Model file for the job. Use its own axes, mm. Face numbers are marked on the shaded views. A direction names the side the tool comes from. Round coordinates to 2 decimals unless told otherwise and drop trailing zeros. Order: outer loops, then holes, each group sorted by start corner. A loop starts at its lowest first (then second) coordinate and runs counter-clockwise, first axis right, second up. Notation, with made-up numbers: (73.5, 28.5) -> (127.5, 28.5) arc R22 ccw to (127.5, 46.5) -> close; hole circle Ø11 at (-24, 74). An arc over 180 degrees is marked (long way). Put each result on its own line as item: value. Start each with the question number.
Q1. Cut at C-C, the plane x = 92. List the corners of the cut face in (y, z).
Q2. Probe L1, parallel to X at y = -3.25, z = 5; L2, parallel to Z at x = 33.5, y = 0; L3, parallel to X at y = 3, z = 1.25. List the from-to ranges inside material, lowest first.
Q3. Cut at D-D, the plane x = 48. List the corners of the cut face in (y, z).
Q4. Cut at A-A, the plane y = 0. List the corners of the cut face in (x, z), and give its area (3 significant figures).
Q5. Flat gauge pins, fed straight in: P1, Ø8, axis at y = 0, z = 0, coming from the -X side; P2, Ø3, axis at x = 4.5, y = -2.5, coming from the -Z side; P3, Ø2, axis at y = -0.5, z = 9, coming from the -X side. Where does each tip first touch, or does it go through?
Q6. 3-axis set-ups, long thin cutter, end or side, ignore diameter. For the marked faces 1, 2, 3 and 4: which of +Z, -Z, +X, -X, +Y, -Y reach the whole face in a straight line?
Q7. Cut at B-B, the plane z = 0. List the corners of the cut face in (x, y).
from build123d import *

# Parameters (mm, degrees)
CHAMFER1_SIZE           = 0.762
SKETCH5_W               = 6.35
SKETCH5_H               = 1.981
CUT_EXTRUDE1_DEPTH      = 10.9185
CUT_EXTRUDE1_DEPTH_BACK = 10.9185
SKETCH6_W               = 6.35
SKETCH6_H               = 1.981
CUT_EXTRUDE2_DEPTH      = 10.9185
CUT_EXTRUDE2_DEPTH_BACK = 10.9185


with BuildPart() as part:
    # Sketch1 → Revolve1 (revolve)
    with BuildSketch(Plane(origin=(0, 0, 0), x_dir=(-1, 0, 0), z_dir=(0, 0, -1)), mode=Mode.PRIVATE) as revolve1_sk:
        with BuildLine():
            Line((-99.4156, 2.774222533), (-99.4156, 0))
            Line((-99.4156, 0), (0, 0))
            Line((0, 0), (0, 9.9185))
            Line((0, 9.9185), (-81.7626, 9.9185))
            Line((-81.7626, 9.9185), (-81.7626, 3.1623))
            Line((-81.7626, 3.1623), (-98.3996, 3.1623))
            ThreePointArc((-98.3996, 3.1623), (-98.943396865, 3.061978675), (-99.4156, 2.774222533))
        make_face()
    revolve(revolve1_sk.sketch.rotate(Axis((99.4156, 0, 0), (-1, 0, 0)), 270), axis=Axis((99.4156, 0, 0), (-1, 0, 0)))  # turned: the seam where the file's is

    # Sketch2 → Cut-Revolve1 (revolve, cut)
    with BuildSketch(Plane(origin=(0, 0, 0), x_dir=(-1, 0, 0), z_dir=(0, 0, -1)), mode=Mode.PRIVATE) as cut_revolve1_sk:
        Polygon((0, 0), (0, 4.953), (-0.127, 4.953), (-0.6604, 4.4196), (-10.5664, 4.4196), (-10.5664, 0), align=None)
    revolve(cut_revolve1_sk.sketch.rotate(Axis((0, 0, 0), (1, 0, 0)), 90), axis=Axis((0, 0, 0), (1, 0, 0)), mode=Mode.SUBTRACT)  # turned: the seam where the file's is

    # Chamfer1
    chamfer1_edges = [part.edges().sort_by_distance(p)[0] for p in [
        (81.7626, 0, -9.9185),
        (0, 0, -9.9185),
    ]]
    chamfer(chamfer1_edges, length=CHAMFER1_SIZE)

    # Sketch5 → Cut-Extrude1 (cut, two sides)
    with BuildSketch(Plane(origin=(0, 0, 0), x_dir=(1, 0, 0), z_dir=(0, 1, 0))) as cut_extrude1_sk:
        with Locations((3.175, 8.928)):
            Rectangle(SKETCH5_W, SKETCH5_H)
        with Locations((3.175, -8.928)):
            Rectangle(SKETCH5_W, SKETCH5_H)
    extrude(amount=CUT_EXTRUDE1_DEPTH, mode=Mode.SUBTRACT)
    extrude(cut_extrude1_sk.sketch, amount=-CUT_EXTRUDE1_DEPTH_BACK, mode=Mode.SUBTRACT)

    # Sketch6 → Cut-Extrude2 (cut, two sides)
    with BuildSketch(Plane(origin=(0, 0, 0), x_dir=(1, 0, 0), z_dir=(0, 1, 0))) as cut_extrude2_sk:
        with Locations((78.5876, 8.928)):
            Rectangle(SKETCH6_W, SKETCH6_H)
        with Locations((78.5876, -8.928)):
            Rectangle(SKETCH6_W, SKETCH6_H)
    extrude(amount=CUT_EXTRUDE2_DEPTH, mode=Mode.SUBTRACT)
    extrude(cut_extrude2_sk.sketch, amount=-CUT_EXTRUDE2_DEPTH_BACK, mode=Mode.SUBTRACT)


solid = part.part
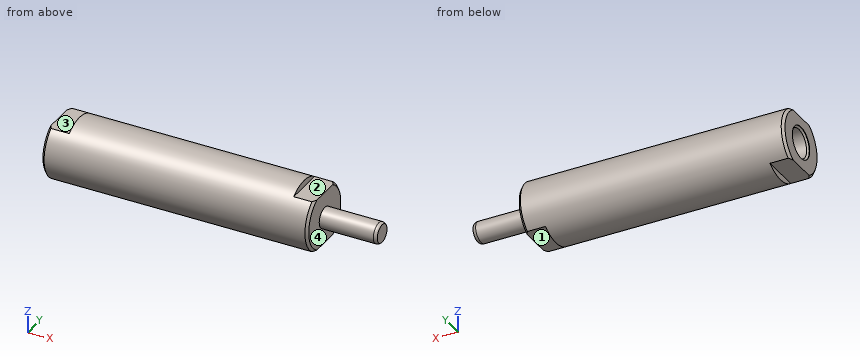
Ans:
1. outline: circle Ø6.32 at (0, 0)
2. L1: x = 0 to 81.76
2. L2: z = -9.92 to 9.92
2. L3: x = 10.57 to 81.76
3. outline: circle Ø19.84 at (0, 0)
4. outline: (0, -7.94) -> (6.35, -7.94) -> (6.35, -9.92) -> (75.41, -9.92) -> (75.41, -7.94) -> (81.76, -7.94) -> (81.76, -3.16) -> (98.4, -3.16) arc R1.52 ccw to (99.42, -2.77) -> (99.42, 2.77) arc R1.52 ccw to (98.4, 3.16) -> (81.76, 3.16) -> (81.76, 7.94) -> (75.41, 7.94) -> (75.41, 9.92) -> (6.35, 9.92) -> (6.35, 7.94) -> (0, 7.94) -> (0, 4.95) -> (0.13, 4.95) -> (0.66, 4.42) -> (10.57, 4.42) -> (10.57, -4.42) -> (0.66, -4.42) -> (0.13, -4.95) -> (0, -4.95) -> close
4. area: 1,590 mm^2
5. P1: stops at x = 10.57
5. P2: stops at z = -7.94
5. P3: stops at x = 6.35
6. face 1: -Z, +X, +Y, -Y
6. face 2: +Z, +X, +Y, -Y
6. face 3: +Z, -X, +Y, -Y
6. face 4: +X
7. outline: (0, -9.16) -> (0.76, -9.92) -> (81, -9.92) -> (81.76, -9.16) -> (81.76, -3.16) -> (98.4, -3.16) arc R1.52 ccw to (99.42, -2.77) -> (99.42, 2.77) arc R1.52 ccw to (98.4, 3.16) -> (81.76, 3.16) -> (81.76, 9.16) -> (81, 9.92) -> (0.76, 9.92) -> (0, 9.16) -> (0, 4.95) -> (0.13, 4.95) -> (0.66, 4.42) -> (10.57, 4.42) -> (10.57, -4.42) -> (0.66, -4.42) -> (0.13, -4.95) -> (0, -4.95) -> close
